from build123d import *

# Parameters (mm, degrees)
BOSS_EXTRUDE1_DEPTH = 4
SKETCH2_R           = 2.5
BOSS_EXTRUDE2_DEPTH = 25


with BuildPart() as part:
    # Sketch1 → Boss-Extrude1 (new body)
    with BuildSketch(Plane.XY):
        Polygon((7.5, 0), (3.75, 6.495190528), (-3.75, 6.495190528), (-7.5, 0), (-3.75, -6.495190528), (3.75, -6.495190528), align=None)
    extrude(amount=BOSS_EXTRUDE1_DEPTH)

    # Sketch2 → Boss-Extrude2 (add)
    with BuildSketch(Plane.XY):
        Circle(SKETCH2_R)
    extrude(amount=-BOSS_EXTRUDE2_DEPTH)

    # Sketch4 → Cut-Revolve1 (revolve, cut)
    with BuildSketch(Plane(origin=(0, 0, 0), x_dir=(0, 0, -1), z_dir=(1, 0, 0)), mode=Mode.PRIVATE) as cut_revolve1_sk:
        with BuildLine():
            Line((-1.722639627, 8.236577674), (-4.518257709, 8.236577674))
            Line((-4.518257709, 8.236577674), (-4.518257709, 5.392544195))
            Line((-4.518257709, 5.392544195), (-4.073554398, 5.392544195))
            ThreePointArc((-4.073554398, 5.392544195), (-3.104166482, 6.984900617), (-1.722639627, 8.236577674))
        make_face()
    revolve(cut_revolve1_sk.sketch.rotate(Axis((0, 0, 0), (0, 0, 1)), 270), axis=Axis((0, 0, 0), (0, 0, 1)), mode=Mode.SUBTRACT)


solid = part.part
Work out the finished part from the listing and answer in its coordinate system (mm). A direction names the side the tool comes from. Give positions to 0.01 mm unless a question says otherwise; leave off trailing zeros. Write each loop counter-clockwise with the first axis right and the second up, starting at its lowest first coordinate (ties: lowest second). Pieces come first, ordered by that corner, then holes. Notation, with made-up numbers: (12.5, 24.5) - (17.5, 24.5) arc R23 cw to (17.5, 49.5) - close; hole circle Ø3 at (66.5, -22.75). An arc over 180 degrees is marked (long way). One line per item, written item: value. Start each with the question number.
1. Given pin 1 (4 mm diameter, centred on y = 4, z = -14.5, fed in from -X); pin 2 (4 mm diameter, centred on y = 3, z = -6.5, fed in from +X); pin 3 (5 mm diameter, centred on x = 4.5, y = 3.5, fed in from -Z), each flat-ended and moving along its own axis, determine where each tip first touches the part or whether it passes through.
2. Consider probe 1 along Z at (x, y) = (1.5, 3); probe 2 along X at (y, z) = (0.25, -5.5); probe 3 along Y at (x, z) = (2.25, -13.25). Determine where each line is inside the solid, lowest interval first.
3. For faces 1 (the cylindrical face through (-0.54, -2.44, -12.32)), 2 (the flat face through (0, 0, -25)), determine the directions among +Z, -Z, +X, -X, +Y, -Y from which every point of the face is accessible in a straight line to the end or side of a thin tool.
4. Find section A-A (z = -5). Write down the section's boundary in (x, y), then the cut area to 3 significant figures.
Geometry results:
1. pin 1: x = -1.5
1. pin 2: x = 2.29
1. pin 3: z = 0
2. probe 1: 0 to 4
2. probe 2: -2.49 to 2.49
2. probe 3: -1.09 to 1.09
3. face 1: -Z
3. face 2: -Z, +X, -X, +Y, -Y
4. outline: circle Ø5 at (0, 0)
4. area: 19.6 mm2
